Model file for the job. Use its own axes, mm. A direction names the side the tool comes from. Round coordinates to 2 decimals unless told otherwise and drop trailing zeros. Order: outer loops, then holes, each group sorted by start corner. A loop starts at its lowest first (then second) coordinate and runs counter-clockwise, first axis right, second up. Notation, with made-up numbers: (-22, -6) -> (-17, -6) arc R27 cw to (-17, 25) -> close; hole circle Ø2 at (53.25, 18). An arc over 180 degrees is marked (long way). Put each result on its own line as item: value. Start each with the question number.
Q1. Probe L1, parallel to Y at x = -7.75, z = -1; L2, parallel to X at y = 8.5, z = -0.5; L3, parallel to Z at x = 8.5, y = -1. List the from-to ranges inside material, lowest first.
Q2. Cut at D-D, the plane y = -2.25. List the corners of the cut face in (x, z), and give its area (3 significant figures).
Q3. Pull direction Y, two halves, no side cores. Call faces 1 (the face through (-9.19, -3.31, -0.99)), 2 (the face through (5.7, 1.3, 0.5)), 3 (the face through (-7.464, 6.308, -0.986)), 4 (the face through (1, 3, 2)): released by +Y, released by -Y, zero draft, split by the parting line, or undercut.
Q4. Flat gauge pins, fed straight in: P1, Ø3, axis at y = 4, z = 3.5, coming from the -X side; P2, Ø4, axis at x = 2, y = 1, coming from the +Z side; P3, Ø5, axis at x = -5, y = 0.5, coming from the +Z side. Where does each tip first touch, or does it go through?
Q5. Cut at C-C, the plane x = -6.5. List the corners of the cut face in (y, z).
Q6. Cut at A-A, the plane x = 0. List the corners of the cut face in (y, z).
Q7. Cut at B-B, the plane y = 9.25. List the corners of the cut face in (x, z).
Q8. 3-axis set-ups, long thin cutter, end or side, ignore diameter. For faces 5 (the face through (-5.7, 0, 0.5)), 6 (the face through (-5.7, -1.3, 0.5)), 7 (the face through (-7.445, -6.292, -0.986)): which of +Z, -Z, +X, -X, +Y, -Y reach the whole face in a straight line?
from build123d import *

# Parameters (mm, degrees)
F1_DEPTH = 2
F5_DEPTH = 1


with BuildPart() as f1:
    # F0 (on Top) → F1 (new body)
    with BuildSketch(Plane.XY):
        Polygon((-6.7911229225, 5.7391721177), (0, 0), (-1.5747073965, 8.7508710698), (-1.8823085464, 10.4602540378), (-8.1176914536, 6.8602540378), align=None)
        with BuildLine():
            Line((-1.5747073965, 8.7508710698), (0, 0))
            Line((0, 0), (1.5747074179, 8.7508711884))
            ThreePointArc((1.5747074179, 8.7508711884), (6.02e-08, 7.4342376439), (-1.5747073965, 8.7508710698))
        make_face()
        Polygon((1.5747074179, 8.7508711884), (0, 0), (6.7911228899, 5.7391720902), (8.1176914536, 6.8602540378), (1.8823085464, 10.4602540378), align=None)
        with BuildLine():
            Line((6.7911228899, 5.7391720902), (0, 0))
            Line((0, 0), (8.3658305386, 3.0116989939))
            ThreePointArc((8.3658305386, 3.0116989939), (6.4382387283, 3.7171186992), (6.7911228899, 5.7391720902))
        make_face()
        Polygon((8.3658305386, 3.0116989939), (0, 0), (8.3658304092, -3.0116989473), (10, -3.6), (10, 3.6), align=None)
        with BuildLine():
            Line((8.3658304092, -3.0116989473), (0, 0))
            Line((0, 0), (6.7911229101, -5.7391721072))
            ThreePointArc((6.7911229101, -5.7391721072), (6.4382386873, -3.7171187701), (8.3658304092, -3.0116989473))
        make_face()
        Polygon((6.7911229101, -5.7391721072), (0, 0), (1.574707395, -8.7508710612), (1.8823085464, -10.4602540378), (8.1176914536, -6.8602540378), align=None)
        with BuildLine():
            Line((1.574707395, -8.7508710612), (0, 0))
            Line((0, 0), (-1.5747073992, -8.7508710849))
            ThreePointArc((-1.5747073992, -8.7508710849), (-1.21e-08, -7.4342376439), (1.574707395, -8.7508710612))
        make_face()
        Polygon((-1.5747073992, -8.7508710849), (0, 0), (-6.791122959, -5.7391721485), (-8.1176914536, -6.8602540378), (-1.8823085464, -10.4602540378), align=None)
        with BuildLine():
            Line((0, 0), (-8.3658303156, -3.0116989136))
            ThreePointArc((-8.3658303156, -3.0116989136), (-6.9038580047, -3.2080883373), (-6.2238793035, -4.517118822))
            ThreePointArc((-6.2238793035, -4.517118822), (-6.3726022536, -5.1907618464), (-6.791122959, -5.7391721485))
            Line((-6.791122959, -5.7391721485), (0, 0))
        make_face()
        Polygon((-8.3658305462, 3.0116989966), (-10, 3.6), (-10, -3.6), (-8.3658303156, -3.0116989136), (0, 0), align=None)
        with BuildLine():
            ThreePointArc((-6.2238793035, 4.517118822), (-6.9038581049, 3.2080882668), (-8.3658305462, 3.0116989966))
            Line((-8.3658305462, 3.0116989966), (0, 0))
            Line((0, 0), (-6.7911229225, 5.7391721177))
            ThreePointArc((-6.7911229225, 5.7391721177), (-6.3726022435, 5.1907618248), (-6.2238793035, 4.517118822))
        make_face()
    extrude(amount=-F1_DEPTH)

    # F2 (on Front) → F3 (revolve)
    with BuildSketch(Plane.XZ):
        with BuildLine():
            Line((-4, 0), (0, 0))
            Line((0, 0), (0, 6))
            ThreePointArc((0, 6), (-2.1213203436, 5.1213203436), (-3, 3))
            Line((-3, 3), (-3, 2))
            Line((-3, 2), (-4, 2))
            Line((-4, 2), (-4, 0))
        make_face()
    revolve(axis=Axis((0, 0, 3), (0, 0, -1)))

    # F4 (on face) → F5 (join)
    with BuildSketch(Plane.XY):
        with BuildLine():
            Line((-3.4071028195, -1.3), (-3.4071028195, 0))
            Line((-3.4071028195, 0), (-4, 0))
            ThreePointArc((-4, 0), (-3.9453405592, -0.6590052141), (-3.7828560639, -1.3))
            Line((-3.7828560639, -1.3), (-3.4071028195, -1.3))
        make_face()
        with BuildLine():
            ThreePointArc((-3.7828560639, -1.3), (-3.9453405592, -0.6590052141), (-4, 0))
            Line((-4, 0), (-7.5, 0))
            Line((-7.5, 0), (-7.5, -1.3))
            Line((-7.5, -1.3), (-3.7828560639, -1.3))
        make_face()
        with BuildLine():
            ThreePointArc((4, 0), (3.9453405592, 0.6590052141), (3.7828560639, 1.3))
            Line((3.7828560639, 1.3), (3.4071028195, 1.3))
            Line((3.4071028195, 1.3), (3.4071028195, 0))
            Line((3.4071028195, 0), (4, 0))
        make_face()
        with BuildLine():
            Line((7.5, 1.3), (3.7828560639, 1.3))
            ThreePointArc((3.7828560639, 1.3), (3.9453405592, 0.6590052141), (4, 0))
            Line((4, 0), (7.5, 0))
            Line((7.5, 0), (7.5, 1.3))
        make_face()
    extrude(amount=F5_DEPTH)


solid = f1.part
Ans:
1. L1: y = -7.07 to -6.55, -2.92 to 2.92, 6.55 to 7.07
1. L2: x = -5.28 to -1.51, 1.51 to 5.28
1. L3: z = -2 to 0
2. outline: (-10, -2) -> (10, -2) -> (10, 0) -> (3.31, 0) -> (3.31, 2) -> (1.98, 2) -> (1.98, 3) arc R1.98 ccw to (-1.98, 3) -> (-1.98, 2) -> (-3.31, 2) -> (-3.31, 0) -> (-10, 0) -> close
2. area: 63.4 mm^2
3. face 1: released by -Y
3. face 2: released by +Y
3. face 3: undercut
3. face 4: zero draft
4. P1: stops at x = -1.61
4. P2: stops at z = 5.99
4. P3: stops at z = 4.62
5. outline: (-7.79, -2) -> (-5.42, -2) -> (-5.42, 0) -> (-7.79, 0) -> close; (-3.62, -2) -> (3.62, -2) -> (3.62, 0) -> (0, 0) -> (0, 1) -> (-1.3, 1) -> (-1.3, 0) -> (-3.62, 0) -> close; (5.42, -2) -> (7.79, -2) -> (7.79, 0) -> (5.42, 0) -> close
6. outline: (-7.43, -2) -> (7.43, -2) -> (7.43, 0) -> (4, 0) -> (4, 2) -> (3, 2) -> (3, 3) arc R3 ccw to (-3, 3) -> (-3, 2) -> (-4, 2) -> (-4, 0) -> (-7.43, 0) -> close
7. outline: (-3.98, -2) -> (-1.66, -2) -> (-1.66, 0) -> (-3.98, 0) -> close; (1.66, -2) -> (3.98, -2) -> (3.98, 0) -> (1.66, 0) -> close
8. face 5: +Z, -X, +Y
8. face 6: +Z, -X, -Y
8. face 7: +Z, -Z, -X
